Read the model definition and answer for the solid it produces. Units are mm, in the model's axes. A direction names the side the tool comes from. Give positions to 0.01 mm unless a question says otherwise; leave off trailing zeros. Loops run counter-clockwise (first coordinate to the right, second up) from the corner with the lowest first, then second, coordinate; pieces in that order, holes last. Notation, with made-up numbers: (-34.5, -1.5) - (-14.5, -1.5) arc R30 cw to (-14.5, 27.5) - close; hole circle Ø8 at (88.5, 17.25). An arc over 180 degrees is marked (long way). Put each result on its own line as item: value. Start each with the question number.
1. A cutting plane is placed at D-D, the plane y = -50. Determine the outline of the cut face in (x, z) (3 decimals), plus the area to 3 significant figures.
2. For a pull along Y with two mould halves and no side action, classify faces 6 (the flat face through (-30.5, -102, 22)), 7 (the flat face through (-14, -44, 2)), 8 (the flat face through (-18.59, -69.24, 2.27)) as released by +Y, released by -Y, zero draft, split by the parting line, or undercut.
3. A cutting plane is placed at B-B, the plane y = -15.5. Determine the outline of the cut face in (x, z).
4. Consider L1, parallel to X at y = -29.5, z = 3; L2, parallel to X at y = -95, z = 2; L3, parallel to Z at x = -12.5, y = -49. Determine where each line is inside the solid, lowest interval first. Write a range as from..to.
5. For faces 1 (the flat face through (-16.5, -20, 2)), 2 (the flat face through (30.5, -102, 22)), 3 (the flat face through (32, -105, 27)), 4 (the flat face through (-30.5, -72, 2)), 5 (the flat face through (-33, -101, 29)), determine the directions among +Z, -Z, +X, -X, +Y, -Y from which every point of the face is accessible in a straight line to the end or side of a thin tool.
6. A cutting plane is placed at C-C, the plane y = -77.5. Determine the outline of the cut face in (x, z), plus the area to 3 significant figures.
7. Given pin 1 Ø1.4 at (y, z) = (-20, 2) entering from -X; pin 2 Ø2.5 at (y, z) = (-25, 2) entering from +X; pin 3 Ø4.5 at (x, z) = (14.5, 2) entering from -Y, each flat-ended and moving along its own axis, determine where each tip first touches the part or whether it passes through.
8. A cutting plane is placed at A-A, the plane z = 15. Determine the outline of the cut face in (x, y).
```python
from build123d import *

# Parameters (mm, degrees)
F1_DEPTH = 4.6
F2_W     = 4
F2_H     = 4
F3_DEPTH = 52
F4_R     = 1.99999


# Not quite as in the source:
# - a fillet or chamfer is up to 0.001 mm smaller than in the source, because OpenCascade refuses the exact size


with BuildPart() as f1:
    # F0 (on Top) → F1 (new body)
    with BuildSketch(Plane.XY):
        Polygon((16.5, 0), (-16.5, 0), (-16.5, -40), (-12.5, -40), (-12.5, -4), (12.5, -4), (12.5, -40), (16.5, -40), align=None)
        Polygon((-12.5, -40), (-16.5, -40), (-18.25, -40), (-34.5, -60), (-34.5, -105), (-30.5, -105), (-30.5, -93.7917722906), (-30.5, -81.420162501), (-30.5, -61.420162501), (-16.346117968, -44), (-12.346117968, -44), (-6.344200027, -44), (6.344200027, -44), (12.346117968, -44), (16.346117968, -44), (30.5, -61.420162501), (30.5, -81.420162501), (30.5, -93.7917722906), (30.5, -105), (34.5, -105), (34.5, -60), (18.25, -40), (16.5, -40), (12.5, -40), align=None)
        Polygon((-30.5, -81.420162501), (-30.5, -93.7917722906), (-6.344200027, -44), (-12.346117968, -44), align=None)
        Polygon((6.344200027, -44), (30.5, -93.7917722906), (30.5, -81.420162501), (12.346117968, -44), align=None)
    extrude(amount=F1_DEPTH)

    # F2 (on face) → F3 (join)
    with BuildSketch(Plane.XY.offset(4.6)):
        with Locations((-32.5, -103)):
            Rectangle(F2_W, F2_H)
        with Locations((32.5, -103)):
            Rectangle(F2_W, F2_H)
    extrude(amount=F3_DEPTH)

    # F4 (radius 2 in the source; OpenCascade refuses exactly that, so slightly less here)
    f4_edges = [f1.edges().sort_by_distance(p)[0] for p in [
        (-32.5, -105, 56.6),
        (-32.5, -101, 56.6),
        (32.5, -105, 56.6),
        (32.5, -101, 56.6),
    ]]
    fillet(f4_edges, radius=F4_R)


solid = f1.part
```
Return value:
1. outline: (-26.375, 0) - (-21.221, 0) - (-21.221, 4.6) - (-26.375, 4.6) - close; (-15.257, 0) - (-9.255, 0) - (-9.255, 4.6) - (-15.257, 4.6) - close; (9.255, 0) - (15.257, 0) - (15.257, 4.6) - (9.255, 4.6) - close; (21.221, 0) - (26.375, 0) - (26.375, 4.6) - (21.221, 4.6) - close
1. area: 103 mm2
2. face 6: zero draft
2. face 7: undercut
2. face 8: released by -Y
3. outline: (-16.5, 0) - (-12.5, 0) - (-12.5, 4.6) - (-16.5, 4.6) - close; (12.5, 0) - (16.5, 0) - (16.5, 4.6) - (12.5, 4.6) - close
4. L1: x = -16.5..-12.5, 12.5..16.5
4. L2: x = -34.5..-30.5, 30.5..34.5
4. L3: z = 0..4.6
5. face 1: +Z, -Z, -X, +Y
5. face 2: +Z, -Z, -Y
5. face 3: +Z, -Z, +X, -X, -Y
5. face 4: +Z, -Z
5. face 5: +Z, +X, -X, +Y
6. outline: (-34.5, 0) - (-30.5, 0) - (-30.5, 4.6) - (-34.5, 4.6) - close; (-28.6, 0) - (-22.6, 0) - (-22.6, 4.6) - (-28.6, 4.6) - close; (22.6, 0) - (28.6, 0) - (28.6, 4.6) - (22.6, 4.6) - close; (30.5, 0) - (34.5, 0) - (34.5, 4.6) - (30.5, 4.6) - close
6. area: 92.0 mm2
7. pin 1: stops at x = -16.5
7. pin 2: stops at x = 16.5
7. pin 3: stops at y = -65.45
8. outline: (-34.5, -105) - (-30.5, -105) - (-30.5, -101) - (-34.5, -101) - close; (30.5, -105) - (34.5, -105) - (34.5, -101) - (30.5, -101) - close
